```python
from build123d import *

# Parameters (mm, degrees)
SKETCH3_R          = 4
SKETCH3_R_2        = 5
CUT_EXTRUDE2_DEPTH = 127.935022748


with BuildPart() as part:
    # Sketch2 → Revolve1 (revolve)
    with BuildSketch(Plane.XY, mode=Mode.PRIVATE) as revolve1_sk:
        Polygon((82.5, 0), (56, 0), (56, 6), (24, 6), (24, 20), (31.256462168, 20), (31.256462168, 50), (41.256462168, 50), (41.256462168, 25), (82.5, 25), align=None)
    revolve(revolve1_sk.sketch.rotate(Axis((0, 0, 0), (0, 1, 0)), 90), axis=Axis((0, 0, 0), (0, 1, 0)))

    # Sketch3 → Cut-Extrude2 (cut, through all)
    with BuildSketch(Plane.XZ):
        with Locations(Location((65, 0, 0), (0, 0, 270))):
            Circle(SKETCH3_R)
        with Locations(Location((45.961940777, -45.961940777, 0), (0, 0, 270))):
            Circle(SKETCH3_R_2)
        with Locations(Location((0, -65, 0), (0, 0, 270))):
            Circle(SKETCH3_R_2)
        with Locations(Location((-45.961940777, -45.961940777, 0), (0, 0, 270))):
            Circle(SKETCH3_R_2)
        with Locations(Location((-65, 0, 0), (0, 0, 270))):
            Circle(SKETCH3_R)
        with Locations(Location((-45.961940777, 45.961940777, 0), (0, 0, 270))):
            Circle(SKETCH3_R)
        with Locations(Location((0, 65, 0), (0, 0, 270))):
            Circle(SKETCH3_R)
        with Locations(Location((45.961940777, 45.961940777, 0), (0, 0, 270))):
            Circle(SKETCH3_R)
    extrude(amount=-CUT_EXTRUDE2_DEPTH, mode=Mode.SUBTRACT)


solid = part.part
```
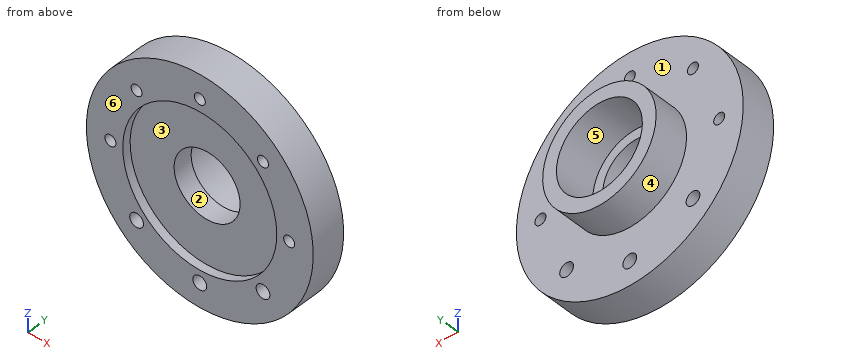
Verification items for the finished model (mm, model axes). Face numbers are marked on the shaded views. A direction names the side the tool comes from. Give positions to 0.01 mm unless a question says otherwise; leave off trailing zeros. Order: outer loops, then holes, each group sorted by start corner. A loop starts at its lowest first (then second) coordinate and runs counter-clockwise, first axis right, second up. Notation, with made-up numbers: (80, 52) - (120, 52) arc R24 cw to (120, 91) - close; hole circle Ø2 at (58, -27.5). An arc over 180 degrees is marked (long way). Answer as CSV lines item,"result". Start each with the question number.
Item 1: Section check A-A, the plane z = 0. Record the boundary of the cut face in (x, y).
Item 2: Gauge pin test, flat ends, axial feed: pin 1 (4 mm diameter, centred on x = 45.5, y = 14, fed in from +Z); pin 2 (1.5 mm diameter, centred on y = 24.5, z = 43.5, fed in from -X); pin 3 (12 mm diameter, centred on y = 13, z = -6.5, fed in from -X); pin 4 (11.5 mm diameter, centred on x = 0, z = -65, fed in from -Y). Record the tip position at first contact, or that the pin passes through.
Item 3: Mould release check, pull along Z, two halves, no side actions. Record for the marked faces 4, 5 and 6: released by +Z, released by -Z, zero draft, split by the parting line, or undercut.
Item 4: Section check C-C, the plane x = 65. Record the boundary of the cut face in (y, z), plus the area to 3 significant figures.
Item 5: Material ranges on L1, parallel to Y at x = -63, z = -37; L2, parallel to X at y = 17, z = -50.5; L3, parallel to Y at x = -12.5, z = 32, recorded low to high.
Item 6: Access from +Z, -Z, +X, -X, +Y, -Y to the whole of each face (thin tool, end or side, straight path). Record for the marked faces 1, 2 and 3.
Item 7: Section check D-D, the plane y = 8.5. State how many separate pieces and enclosed holes the cut face has, plus the area to 3 significant figures.
Item 8: Section check B-B, the plane x = 0. Record the boundary of the cut face in (y, z), plus the area to 3 significant figures.
Filled in:
1,outline,"(-82.5, 0) - (-69, 0) - (-69, 25) - (-82.5, 25) - close; (-61, 0) - (-56, 0) - (-56, 6) - (-24, 6) - (-24, 20) - (-31.26, 20) - (-31.26, 50) - (-41.26, 50) - (-41.26, 25) - (-61, 25) - close; (24, 6) - (56, 6) - (56, 0) - (61, 0) - (61, 25) - (41.26, 25) - (41.26, 50) - (31.26, 50) - (31.26, 20) - (24, 20) - close; (69, 0) - (82.5, 0) - (82.5, 25) - (69, 25) - close"
2,pin 1,"z = 70.1"
2,pin 2,"x = -70.56"
2,pin 3,"x = -82.5"
2,pin 4,"y = 0"
3,face 4,"split by the parting line"
3,face 5,"undercut"
3,face 6,"zero draft"
4,outline,"(0, -50.81) - (25, -50.81) - (25, -4) - (0, -4) - close; (0, 4) - (25, 4) - (25, 50.81) - (0, 50.81) - close"
4,area,"2,340 mm^2"
5,L1,"0 to 25"
5,L2,"-65.24 to -48.06, -43.86 to 43.86, 48.06 to 65.24"
5,L3,"6 to 50"
6,face 1,"+Y"
6,face 2,"+Y, -Y"
6,face 3,"-Y"
7,separate pieces,"1"
7,enclosed holes,"9"
7,area,"19,100 mm^2"
8,outline,"(0, -82.5) - (25, -82.5) - (25, -70) - (0, -70) - close; (0, -60) - (25, -60) - (25, -41.26) - (50, -41.26) - (50, -31.26) - (20, -31.26) - (20, -24) - (6, -24) - (6, -56) - (0, -56) - close; (0, 56) - (6, 56) - (6, 24) - (20, 24) - (20, 31.26) - (50, 31.26) - (50, 41.26) - (25, 41.26) - (25, 61) - (0, 61) - close; (0, 69) - (25, 69) - (25, 82.5) - (0, 82.5) - close"
8,area,"2,520 mm^2"
